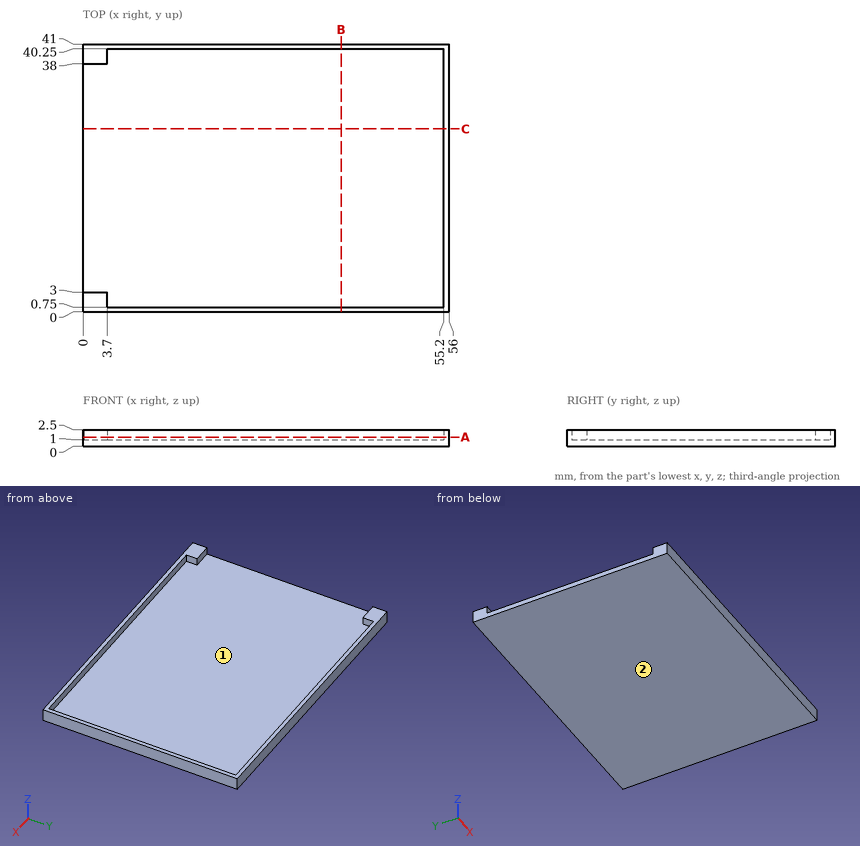
Check sheet for the drawn part. Datum: minimum x, y, z corner. Units: mm. Coordinates: 2 decimals unless noted, no trailing zeros. Order: outer loops, then holes, each group sorted by start corner. A loop starts at its lowest first (then second) coordinate and runs counter-clockwise, first axis right, second up. Notation, with made-up numbers: (-29.5, 26.5) -> (22.5, 26.5) arc R5 cw to (22.5, 31.5) -> close; hole circle Ø6 at (-8.75, 80.5). An arc over 180 degrees is marked (long way). Write each question's results on one line, items separated by ' | '. Start each with the question number.
1) Draft check along Y on the marked faces 1 and 2. Enter one of: pulls with the +Y half, pulls with the -Y half, needs draft (parallel to the pull), parting line crosses it, or undercut.
2) Section check C-C (y = 28). Enter the section's corners in (x, z).
3) Section check A-A (z = 1.4). Enter the section's corners in (x, y).
4) Material ranges on line 1 along Y through (x, z) = (34, 1.55); line 2 along X through (y, z) = (15, 1.65); line 3 along Z through (x, y) = (36, 16), recorded low to high.
5) Depth check by flat-ended pin: pin 1 (10 mm diameter, centred on x = 27.5, y = 35.5, fed in from +Z); pin 2 (6 mm diameter, centred on x = 12.5, y = 11.5, fed in from +Z). Enter the tip coordinate at first touch or a pass-through.
6) Section check B-B (x = 39.5). Enter the section's corners in (y, z), and give its area (4 significant figures).
Checked values:
1) face 1: undercut | face 2: needs draft
2) outline: (0, 0) -> (56, 0) -> (56, 2.5) -> (55.2, 2.5) -> (55.2, 1) -> (0, 1) -> close
3) outline: (0, 0) -> (56, 0) -> (56, 41) -> (0, 41) -> (0, 38) -> (3.7, 38) -> (3.7, 40.25) -> (55.2, 40.25) -> (55.2, 0.75) -> (3.7, 0.75) -> (3.7, 3) -> (0, 3) -> close
4) line 1: 0 to 0.75, 40.25 to 41 | line 2: 55.2 to 56 | line 3: 0 to 1
5) pin 1: z = 2.5 | pin 2: z = 1
6) outline: (0, 0) -> (41, 0) -> (41, 2.5) -> (40.25, 2.5) -> (40.25, 1) -> (0.75, 1) -> (0.75, 2.5) -> (0, 2.5) -> close | area: 43.25 mm²
